from build123d import *

# Parameters (mm, degrees)
F0_W     = 400
F0_H     = 400
F0_R     = 5
F0_R_2   = 2.5
F1_DEPTH = 5


with BuildPart() as f1:
    # F0 (on Top) → F1 (new body)
    with BuildSketch(Plane.XY):
        Rectangle(F0_W, F0_H)
        with Locations((0, -180)):
            Circle(F0_R, mode=Mode.SUBTRACT)
        with Locations((0, -137)):
            Circle(F0_R_2, mode=Mode.SUBTRACT)
        with Locations((-180, 0)):
            Circle(F0_R, mode=Mode.SUBTRACT)
        with Locations((-137, 0)):
            Circle(F0_R_2, mode=Mode.SUBTRACT)
        Circle(F0_R, mode=Mode.SUBTRACT)
        with Locations((137, 0)):
            Circle(F0_R_2, mode=Mode.SUBTRACT)
        with Locations((180, 0)):
            Circle(F0_R, mode=Mode.SUBTRACT)
        with Locations((0, 137)):
            Circle(F0_R_2, mode=Mode.SUBTRACT)
        with Locations((0, 180)):
            Circle(F0_R, mode=Mode.SUBTRACT)
    extrude(amount=F1_DEPTH)


solid = f1.part
Geometry check sheet. Reference: the model listing, model coordinates, mm. Give positions to 0.01 mm unless a question says otherwise; leave off trailing zeros. Loops run counter-clockwise (first coordinate to the right, second up) from the corner with the lowest first, then second, coordinate; pieces in that order, holes last. Notation, with made-up numbers: (56, 44.25) -> (97, 44.25) arc R24 ccw to (97, 76.25) -> close; hole circle Ø6 at (-11, -40). An arc over 180 degrees is marked (long way). Answer in a Markdown table with one row per item. Add a question column.
1) Draft check along X on faces 1 (the face through (-0.651, 184.957, 2.465)), 2 (the face through (42, 3, 5)). Enter one of: pulls with the +X half, pulls with the -X half, needs draft (parallel to the pull), parting line crosses it, or undercut.
2) Cross-section at A-A on x = 180. Record the boundary of the cut face in (y, z).
3) Material ranges on probe 1 along Y at (x, z) = (0, 1.95); probe 2 along Y at (x, z) = (137, 3.6); probe 3 along Y at (x, z) = (-183, 1.05), recorded low to high. Write a range as from..to.
Outcome:
| question | item | result |
|---|---|---|
| 1 | face 1 | undercut |
| 1 | face 2 | needs draft |
| 2 | outline | (-200, 0) -> (-5, 0) -> (-5, 5) -> (-200, 5) -> close; (5, 0) -> (200, 0) -> (200, 5) -> (5, 5) -> close |
| 3 | probe 1 | y = -200..-185, -175..-139.5, -134.5..-5, 5..134.5, 139.5..175, 185..200 |
| 3 | probe 2 | y = -200..-2.5, 2.5..200 |
| 3 | probe 3 | y = -200..-4, 4..200 |
